The figure shows three views and two pictorial views of one solid part (mm, origin at its lowest corner). Answer the questions. Coordinates: 2 decimals unless noted, no trailing zeros. Order: outer loops, then holes, each group sorted by start corner. A loop starts at its lowest first (then second) coordinate and runs counter-clockwise, first axis right, second up. Notation, with made-up numbers: (8, 44.25) -> (61, 44.25) arc R34 cw to (61, 83.25) -> close; hole circle Ø10 at (72, 6). An arc over 180 degrees is marked (long way). Write item = value, one per line. Start each with the question number.
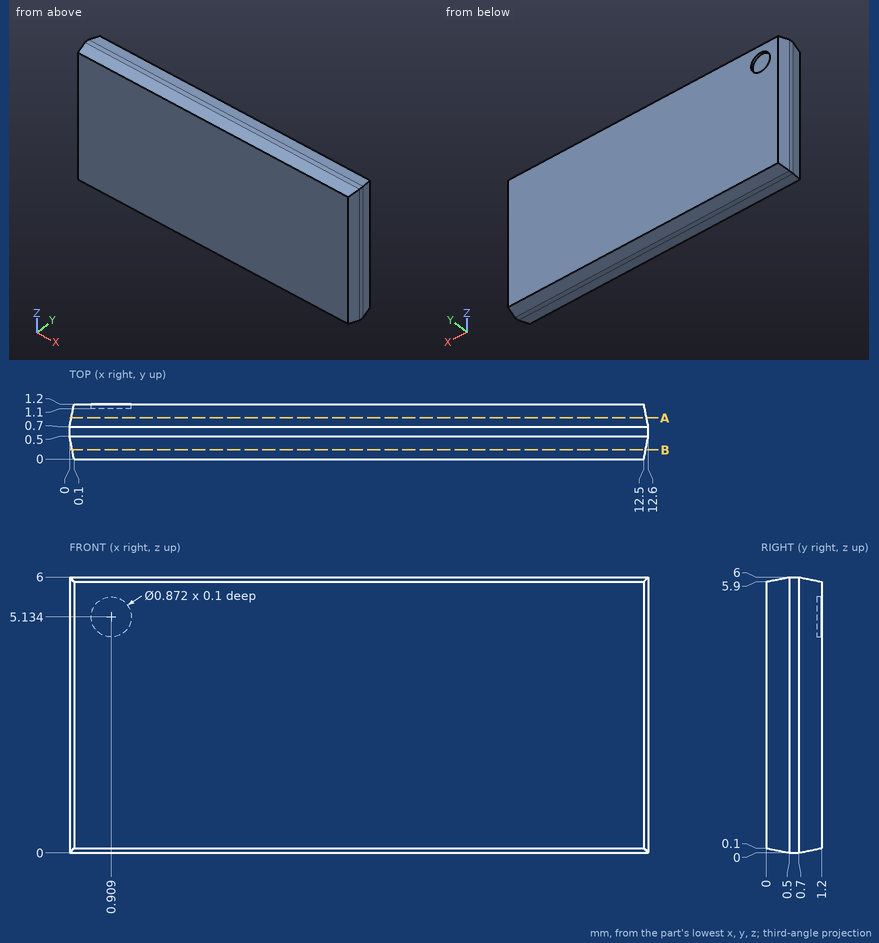
Item 1: Consider probe 1 along X at (y, z) = (0.9, 3.3); probe 2 along X at (y, z) = (1.1, 3.6); probe 3 along Z at (x, y) = (7.5, 0.35). Determine where each line is inside the solid, lowest interval first.
Item 2: Section A-A, the plane y = 0.9 is taken. Give the vertices of the cut face in (x, z).
Item 3: Section B-B, the plane y = 0.2 is taken. Give the vertices of the cut face in (x, z).
A:
q1.probe_1 = 0.04 to 12.56
q1.probe_2 = 0.08 to 12.52
q1.probe_3 = 0.03 to 5.97
q2.outline = (0.04, 0.04) -> (12.56, 0.04) -> (12.56, 5.96) -> (0.04, 5.96) -> close
q3.outline = (0.06, 0.06) -> (12.54, 0.06) -> (12.54, 5.94) -> (0.06, 5.94) -> close
